from build123d import *

# Parameters (mm, degrees)
F0_R          = 1
F2_DEPTH      = 15
F3_DEPTH      = 15.001
F5_DEPTH      = 5.001
F5_DEPTH_BACK = 5.001


with BuildPart() as f2:
    # F0 (on Top) → F2 (new body)
    with BuildSketch(Plane.XY):
        with BuildLine():
            ThreePointArc((-5, 8.0777472107), (-4.6233105022, -8.2990963363), (9.5, 0))
            ThreePointArc((9.5, 0), (8.2990963363, 4.6233105022), (5, 8.0777472107))
            ThreePointArc((5, 8.0777472107), (0, 9.5), (-5, 8.0777472107))
        make_face()
        with BuildLine():
            ThreePointArc((-5, 8.0777472107), (0, 9.5), (5, 8.0777472107))
            ThreePointArc((5, 8.0777472107), (0, 12.2076506099), (-5, 8.0777472107))
        make_face()
        with Locations((0, 10.8538253049)):
            Circle(F0_R, mode=Mode.SUBTRACT)
    extrude(amount=F2_DEPTH)

    # F1 (on Top) → F3 (cut, through all)
    with BuildSketch(Plane.XY):
        with BuildLine():
            Line((-5, 0), (0, 0))
            Line((0, 0), (5, 0))
            Line((5, 0), (5, 8.0777472107))
            ThreePointArc((5, 8.0777472107), (0, 9.5), (-5, 8.0777472107))
            Line((-5, 8.0777472107), (-5, 0))
        make_face()
        with BuildLine():
            Line((5, 0), (0, 0))
            Line((0, 0), (-5, 0))
            Line((-5, 0), (-5, 8.0777472107))
            ThreePointArc((-5, 8.0777472107), (-4.6233105022, -8.2990963363), (9.5, 0))
            ThreePointArc((9.5, 0), (8.2990963363, 4.6233105022), (5, 8.0777472107))
            Line((5, 8.0777472107), (5, 0))
        make_face()
        with BuildLine():
            Line((5, 20), (5, 8.0777472107))
            ThreePointArc((5, 8.0777472107), (8.2990963363, 4.6233105022), (9.5, 0))
            ThreePointArc((9.5, 0), (-4.6233105022, -8.2990963363), (-5, 8.0777472107))
            Line((-5, 8.0777472107), (-5, 20))
            Line((-5, 20), (-15, 20))
            Line((-15, 20), (-15, -15))
            Line((-15, -15), (15, -15))
            Line((15, -15), (15, 20))
            Line((15, 20), (5, 20))
        make_face()
    extrude(amount=F3_DEPTH, mode=Mode.SUBTRACT)

    # F4 (on Right) → F5 (cut, two sides)
    with BuildSketch(Plane.YZ) as f5_sk:
        Polygon((17.0873440802, 4.1219498962), (0, 0), (17.0873440802, 0), align=None)
    extrude(amount=F5_DEPTH, mode=Mode.SUBTRACT)
    extrude(f5_sk.sketch, amount=-F5_DEPTH_BACK, mode=Mode.SUBTRACT)


solid = f2.part
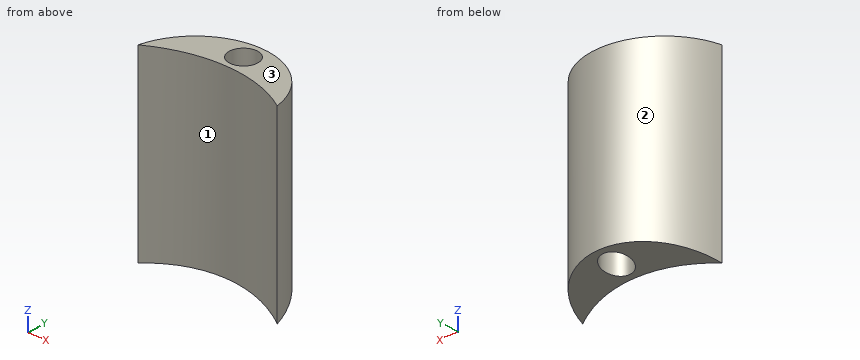
The listing builds one solid part. Answer for the finished solid, in the listing's coordinates (mm). Face numbers are marked on the shaded views. Coordinates: 2 decimals unless noted, no trailing zeros. Loops run counter-clockwise (first coordinate to the right, second up) from the corner with the lowest first, then second, coordinate; pieces in that order, holes last. Notation, with made-up numbers: (37.5, 77.5) -> (65.5, 77.5) arc R19 cw to (65.5, 92.5) -> close; hole circle Ø4 at (53, 18.5). An arc over 180 degrees is marked (long way). Write item = value, one per line. Start each with the question number.
1) A cutting plane is placed at B-B (x = 0). Give the vertices of the cut face in (y, z), then the cut area to 3 significant figures.
2) The mould has two halves that part along X. Classify the marked faces 1, 2 and 3: released by +X, released by -X, zero draft, split by the parting line, or undercut.
3) A cutting plane is placed at D-D (x = -2.25). Give the vertices of the cut face in (y, z).
4) A cutting plane is placed at C-C (z = 7.75). Give the vertices of the cut face in (x, y), then the cut area to 3 significant figures.
5) Straight lines are drawn through the part: line 1 (Y direction, x = 0, z = 9); line 2 (X direction, y = 10.05, z = 3.5); line 3 (X direction, y = 10.4, z = 12.75). For each, find the intervals that lie inside material, in ascending order. Write a range as from..to.
6) Given pin 1 Ø1.5 at (y, z) = (10.5, 3.5) entering from +X; pin 2 Ø5 at (x, z) = (0.5, 9.5) entering from +Y; pin 3 Ø1 at (y, z) = (9, 5.5) entering from +X, each flat-ended and moving along its own axis, determine where each tip first touches the part or whether it passes through.
7) A cutting plane is placed at A-A (y = 10.55). Give the vertices of the cut face in (x, z).
Responses:
q1.outline = (9.5, 2.29) -> (9.85, 2.38) -> (9.85, 15) -> (9.5, 15) -> close; (11.85, 2.86) -> (12.21, 2.94) -> (12.21, 15) -> (11.85, 15) -> close
q1.area = 8.76 mm²
q2.face_1 = undercut
q2.face_2 = split by the parting line
q2.face_3 = zero draft
q3.outline = (9.23, 2.23) -> (11.68, 2.82) -> (11.68, 15) -> (9.23, 15) -> close
q4.outline = (-5, 8.08) arc R9.5 cw to (5, 8.08) arc R5.09 ccw to start; hole circle Ø2 at (0, 10.85)
q4.area = 18.2 mm²
q5.line_1 = 9.5..9.85, 11.85..12.21
q5.line_2 = -4.16..-0.59, 0.59..4.16
q5.line_3 = -3.89..-0.89, 0.89..3.89
q6.pin_1 = 4.36
q6.pin_2 = 12.21
q6.pin_3 = 4.9
q7.outline = (-3.76, 2.54) -> (-0.95, 2.54) -> (-0.95, 15) -> (-3.76, 15) -> close; (0.95, 2.54) -> (3.76, 2.54) -> (3.76, 15) -> (0.95, 15) -> close
